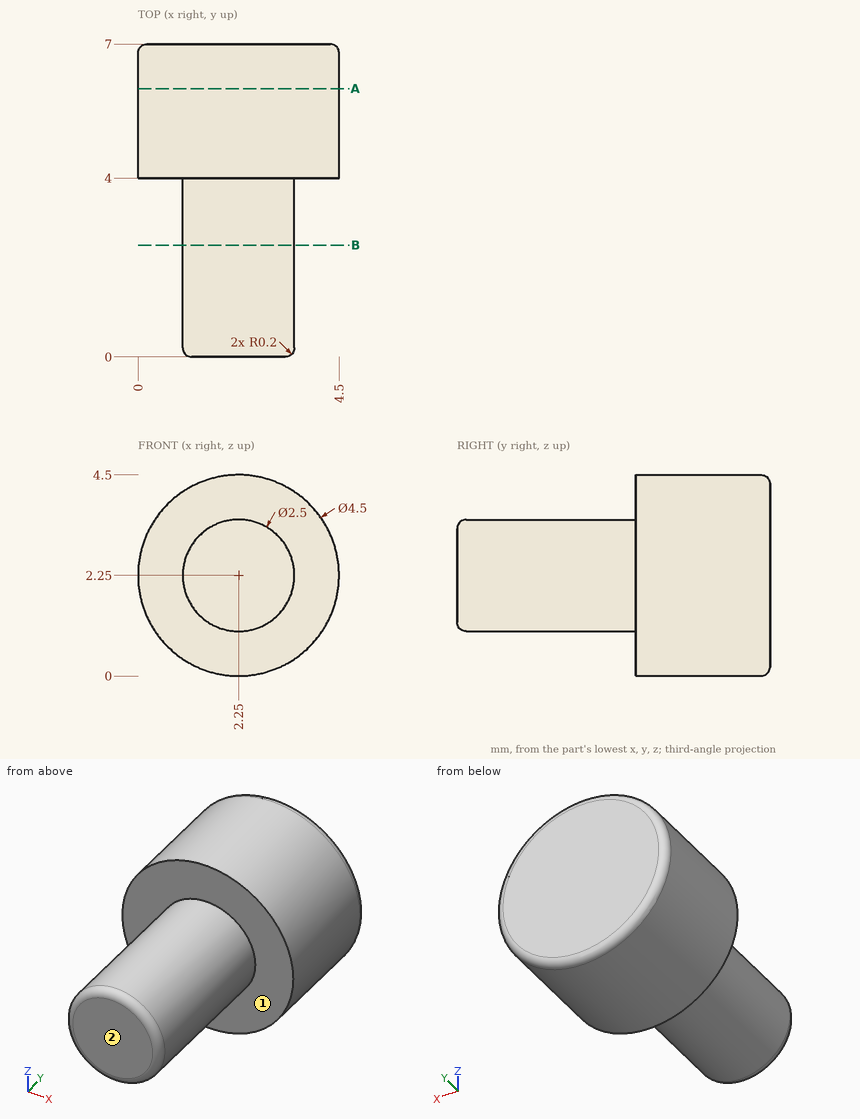
Geometry check sheet. Reference: drawing and pictorial views, mm from the part's lowest x, y, z. A direction names the side the tool comes from. Coordinates: 2 decimals unless noted, no trailing zeros. Write each loop counter-clockwise with the first axis right and the second up, starting at its lowest first coordinate (ties: lowest second). Pieces come first, ordered by that corner, then holes. Notation, with made-up numbers: (18, 14.25) - (61, 14.25) arc R8 cw to (61, 23.25) - close; hole circle Ø1 at (-28.75, 14.25). An arc over 180 degrees is marked (long way). Write item = value, one per line.
Q1. Access from +Z, -Z, +X, -X, +Y, -Y to the whole of each face (thin tool, end or side, straight path). Record for the marked faces 1 and 2.
Answer:
face_1 = -Y
face_2 = +Z, -Z, +X, -X, -Y
Q2. Cross-section at B-B (y = 2.5). Enter the section's corners in (x, z).
Answer:
outline = circle Ø2.5 at (2.25, 2.25)
Q3. Material ranges on L1, parallel to Y at x = 3.4, z = 3.4; L2, parallel to Z at x = 1.3, y = 3; L3, parallel to Z at x = 1.7, y = 6.5, recorded low to high. Write a range as from..to.
Answer:
L1 = 4..7
L2 = 1.44..3.06
L3 = 0.07..4.43
Q4. Cross-section at A-A (y = 6). Enter the section's corners in (x, z), plus the area to 3 significant figures.
Answer:
outline = circle Ø4.5 at (2.25, 2.25)
area = 15.9 mm²
